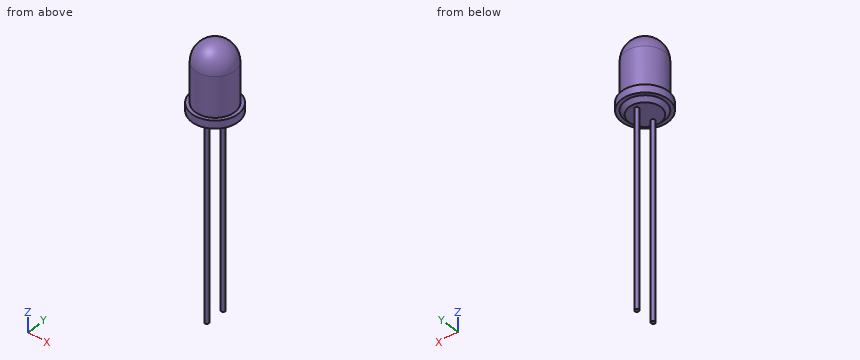
```python
from build123d import *

# Parameters (mm, degrees)
SKETCH_1_R      = 2.5
EXTRUDE_1_DEPTH = 7.6
FILLET_1_R      = 2.5
SKETCH_2_R      = 2.95
EXTRUDE_2_DEPTH = 1
EXTRUDE_START   = 0.5
SKETCH_3_R      = 2.5
EXTRUDE_3_DEPTH = 0.5
CHAMFER_1_SIZE  = 0.5
SKETCH_4_R      = 0.25
EXTRUDE_4_DEPTH = 25


with BuildPart() as part:
    # Эскиз1 → Бобышка-Вытянуть1 (new body)
    with BuildSketch(Plane.XY):
        with Locations(Location((0, 0, 0), (0, 0, 180))):
            Circle(SKETCH_1_R)
    extrude(amount=EXTRUDE_1_DEPTH)

    # Скругление1
    fillet_1_edges = [part.edges().sort_by_distance(p)[0] for p in [
        (2.5, 0, 7.6),
    ]]
    fillet(fillet_1_edges, radius=FILLET_1_R)

    # Эскиз2 → Бобышка-Вытянуть2 (add)
    with BuildSketch(Plane(origin=(0, 0, 0), x_dir=(-1, 0, 0), z_dir=(0, 0, -1))):
        Circle(SKETCH_2_R)
    extrude(amount=EXTRUDE_2_DEPTH)

    # Эскиз3 → Бобышка-Вытянуть3 (add)
    with BuildSketch(Plane(origin=(0, 0, -1), x_dir=(-1, 0, 0), z_dir=(0, 0, -1)).offset(EXTRUDE_START)):
        Circle(SKETCH_3_R)
    extrude(amount=-EXTRUDE_3_DEPTH)

    # Фаска1
    chamfer_1_edges = [part.edges().sort_by_distance(p)[0] for p in [
        (2.5, 0, -1.5),
    ]]
    chamfer(chamfer_1_edges, length=CHAMFER_1_SIZE - 0.0001)  # a hair under: the kernel refuses the full size

    # Эскиз4 → Бобышка-Вытянуть4 (add)
    with BuildSketch(Plane(origin=(0, 0, -1.5), x_dir=(-1, 0, 0), z_dir=(0, 0, -1))):
        with Locations((0, 1.27)):
            Circle(SKETCH_4_R)
        with Locations((0, -1.27)):
            Circle(SKETCH_4_R)
    extrude(amount=EXTRUDE_4_DEPTH)


solid = part.part
```
Read the model definition and answer for the solid it produces. Units are mm, in the model's axes. Give positions to 0.01 mm unless a question says otherwise; leave off trailing zeros. Loops run counter-clockwise (first coordinate to the right, second up) from the corner with the lowest first, then second, coordinate; pieces in that order, holes last.
Item 1: The part is cut by section A-A (z = -22). Write down the section's boundary in (x, y).
Item 2: Find the intervals of material crossed by line 1 along Z through (x, y) = (1.2, -2.35); line 2 along Y through (x, z) = (0, -24); line 3 along X through (y, z) = (-0.1, 3.5), in increasing order.
Item 3: Each of these flat-tipped pins is pushed along its axis until it touches: pin 1 Ø2 at (x, y) = (-2, 0) entering from -Z; pin 2 Ø1.5 at (x, y) = (-1.5, -2) entering from +Z; pin 3 Ø3 at (y, z) = (-0.5, 3) entering from +X. Where does it stop, or does it pass through?
Taken from the geometry:
1. outline: circle Ø0.5 at (0, -1.27); circle Ø0.5 at (0, 1.27)
2. line 1: z = -1 to 0
2. line 2: y = -1.52 to -1.02, 1.02 to 1.52
2. line 3: x = -2.5 to 2.5
3. pin 1: stops at z = -1.5
3. pin 2: stops at z = 6.89
3. pin 3: stops at x = 2.5
